Build history of the part. All positions in model axes, mm. Face numbers are marked on the shaded views. A direction names the side the tool comes from. Give positions to 0.01 mm unless a question says otherwise; leave off trailing zeros. Loops run counter-clockwise (first coordinate to the right, second up) from the corner with the lowest first, then second, coordinate; pieces in that order, holes last. Notation, with made-up numbers: (79, 72.25) -> (109, 72.25) arc R28 cw to (109, 103.25) -> close; hole circle Ø3 at (62.5, -24.5). An arc over 180 degrees is marked (long way). Answer in a Markdown table with one row per item. Add a question column.
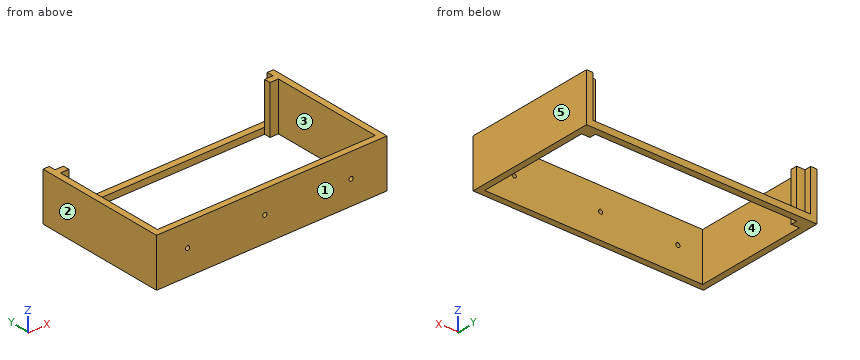
from build123d import *

# Parameters (mm, degrees)
F0_R      = 8
F1_DEPTH  = 3
F2_W      = 3
F2_H      = 3
F2_W_2    = 104
F3_DEPTH  = 20
F4_W      = 3
F4_H      = 20
F5_DEPTH  = 104.4
F6_W      = 96
F6_H      = 3
F7_DEPTH  = 40
F8_R      = 1.5
F9_DEPTH  = 3
F10_R     = 8
F12_DEPTH = 40
F13_R     = 1
F14_DEPTH = 3


with BuildPart() as f1:
    # F0 (on Top) → F1 (new body)
    with BuildSketch(Plane.XY):
        Polygon((-40, 33.034884), (-50, 33.034884), (-50, 18.034884), (-50, 0.034884), (-50, -2.965116), (-50, -17.965116), (-50, -29.965116), (60, -29.965116), (60, -24.965116), (60, -14.965116), (60, -9.965116), (60, -4.965116), (60, 0.034884), (60, 18.034884), (60, 33.034884), (40, 33.034884), (20, 33.034884), (0, 33.034884), (-20, 33.034884), align=None)
        with Locations((25, -0.468963)):
            Circle(F0_R, mode=Mode.SUBTRACT)
        with Locations((-15, 1.034884)):
            Circle(F0_R, mode=Mode.SUBTRACT)
    extrude(amount=F1_DEPTH)

    # F2 (on face) → F3 (join)
    with BuildSketch(Plane.XY.offset(3)):
        with Locations((-48.5, -28.465116)):
            Rectangle(F2_W, F2_H)
        with Locations((5, -28.465116)):
            Rectangle(F2_W_2, F2_H)
        Polygon((-50, 30.034884), (-50, -26.965116), (-47, -26.965116), (-47, 33.034884), (-50, 33.034884), align=None)
        with Locations((58.5, -28.465116)):
            Rectangle(F2_W, F2_H)
        Polygon((57, 33.034884), (57, -26.965116), (60, -26.965116), (60, 30.034884), (60, 33.034884), align=None)
    extrude(amount=F3_DEPTH)

    # F4 (on face) → F5 (join)
    with BuildSketch(Plane.YZ.offset(-47)):
        with Locations((28.334884, 13)):
            Rectangle(F4_W, F4_H)
    extrude(amount=F5_DEPTH)

    # F6 (on face) → F7 (cut)
    with BuildSketch(Plane.XY.offset(23)):
        with Locations((5, 28.334884)):
            Rectangle(F6_W, F6_H)
    extrude(amount=-F7_DEPTH, mode=Mode.SUBTRACT)

    # F8 (on face) → F9 (cut)
    with BuildSketch(Plane(origin=(0, -26.965116, 0), x_dir=(-1, 0, 0), z_dir=(0, 1, 0))):
        with Locations((17, 26.988985)):
            Circle(F8_R)
        with Locations((-27, 26.988985)):
            Circle(F8_R)
        with Locations((-20, 26.988985)):
            Circle(F8_R)
    extrude(amount=-F9_DEPTH, mode=Mode.SUBTRACT)

    # F10 (on face) → F12 (cut)
    with BuildSketch(Plane.XY.offset(3)):
        Polygon((53, 26.834884), (-43, 26.834884), (-47, 26.834884), (-47, -26.965116), (57, -26.965116), (57, 26.834884), align=None)
        with Locations((25, -0.468963)):
            Circle(F10_R, mode=Mode.SUBTRACT)
        with Locations((-15, 1.034884)):
            Circle(F10_R, mode=Mode.SUBTRACT)
    extrude(amount=-F12_DEPTH, mode=Mode.SUBTRACT)

    # F13 (on face) → F14 (cut)
    with BuildSketch(Plane.XZ.offset(29.965116)):
        with Locations((-35.19102, 12.040687)):
            Circle(F13_R)
        with Locations((1.695728, 12.003587)):
            Circle(F13_R)
        with Locations((42.899329, 11.5)):
            Circle(F13_R)
    extrude(amount=-F14_DEPTH, mode=Mode.SUBTRACT)


solid = f1.part
(1) Saw through at C-C, the plane z = 17.25. List the corners of the cut face in (x, y).
(2) Saw through at B-B, the plane x = 48.5. List the corners of the cut face in (y, z).
(3) Flat gauge pins, fed straight in: pin 1 Ø3.5 at (x, y) = (-20.5, 31.5) entering from +Z; pin 2 Ø1.2 at (x, z) = (56, 15) entering from +Y; pin 3 Ø2.5 at (x, z) = (42.9, 11.5) entering from +Y; pin 4 Ø1.6 at (x, z) = (-35.19, 12.04) entering from -Y. Where does each tip first touch, or does it go through?
(4) Saw through at A-A, the plane y = 0. List the corners of the cut face in (x, z), then the cut area to 3 significant figures.
(5) Wall check: line 1 along X through (y, z) = (20.5, 7.25); line 2 along X through (y, z) = (29.5, 21.5); line 3 along Y through (x, z) = (20, 6.25). Give the ranges that are in metal, low to high. Write a range as from..to.
(6) Two-plate mould, pull along Y, no slides. Class the marked faces 1, 2 and 3: released by +Y, released by -Y, zero draft, split by the parting line, or undercut.
(7) 3-axis set-ups, long thin cutter, end or side, ignore diameter. For the marked faces 4 and 5: which of +Z, -Z, +X, -X, +Y, -Y reach the whole face in a straight line?
Worked answers:
| question | item | result |
|---|---|---|
| 1 | outline | (-50, -29.97) -> (60, -29.97) -> (60, 33.03) -> (57, 33.03) -> (57, 29.83) -> (53, 29.83) -> (53, 26.83) -> (57, 26.83) -> (57, -26.97) -> (-47, -26.97) -> (-47, 26.83) -> (-43, 26.83) -> (-43, 29.83) -> (-47, 29.83) -> (-47, 33.03) -> (-50, 33.03) -> close |
| 2 | outline | (-29.97, 0) -> (-26.97, 0) -> (-26.97, 23) -> (-29.97, 23) -> close; (29.83, 0) -> (33.03, 0) -> (33.03, 3) -> (29.83, 3) -> close |
| 3 | pin 1 | z = 3 |
| 3 | pin 2 | y = 29.83 |
| 3 | pin 3 | y = -26.97 |
| 3 | pin 4 | through |
| 4 | outline | (-50, 0) -> (-47, 0) -> (-47, 23) -> (-50, 23) -> close; (57, 0) -> (60, 0) -> (60, 23) -> (57, 23) -> close |
| 4 | area | 138 mm^2 |
| 5 | line 1 | -50..-47, 57..60 |
| 5 | line 2 | -50..-43, 53..60 |
| 5 | line 3 | -29.97..-26.97 |
| 6 | face 1 | released by -Y |
| 6 | face 2 | zero draft |
| 6 | face 3 | undercut |
| 7 | face 4 | +Z, -Z |
| 7 | face 5 | +Z, -Z, +X, +Y, -Y |
